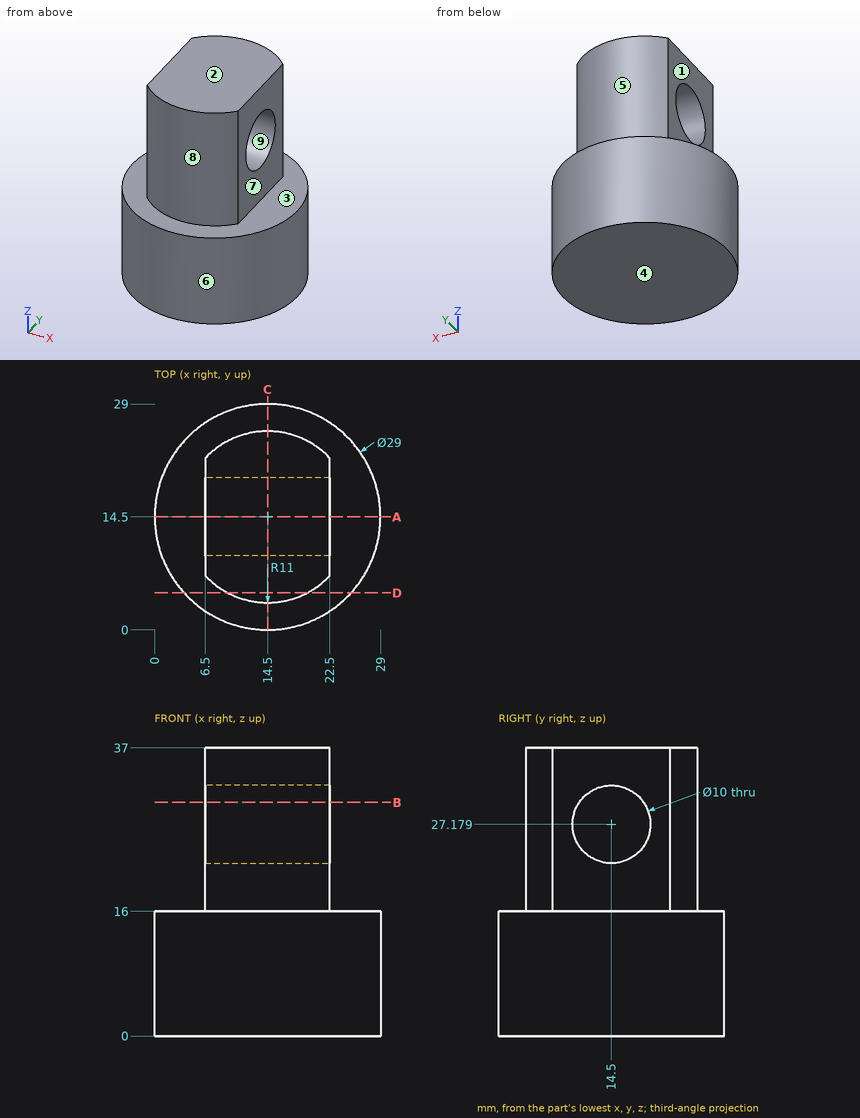
Geometry check sheet. Reference: drawing and pictorial views, mm from the part's lowest x, y, z. A direction names the side the tool comes from. Coordinates: 2 decimals unless noted, no trailing zeros. Loops run counter-clockwise (first coordinate to the right, second up) from the corner with the lowest first, then second, coordinate; pieces in that order, holes last.
1) Sectioned sample at B-B (z = 30). Record the boundary of the cut face in (x, y), and give its area (3 significant figures).
2) Release check for a two-part mould opening along Y. For the marked faces 6, 7, 8 and 9 record: released by +Y, released by -Y, zero draft, split by the parting line, or undercut.
3) Access from +Z, -Z, +X, -X, +Y, -Y to the whole of each face (thin tool, end or side, straight path). Record for the marked faces 1, 2, 3, 4 and 5.
4) Material ranges on probe 1 along Z at (x, y) = (14.75, 14.5); probe 2 along Z at (x, y) = (12, 2); probe 3 along X at (y, z) = (8.5, 18), recorded low to high.
5) Gauge pin test, flat ends, axial feed: pin 1 (2 mm diameter, centred on x = 10.5, z = 9.5, fed in from -Y); pin 2 (4 mm diameter, centred on x = 24.5, z = 5, fed in from -Y); pin 3 (3 mm diameter, centred on y = 11, z = 13, fed in from +X). Record the tip position at first contact, or that the pin passes through.
6) Sectioned sample at D-D (y = 4.75). Record the boundary of the cut face in (x, z).
7) Sectioned sample at C-C (x = 14.5). Record the boundary of the cut face in (y, z).
8) Sectioned sample at A-A (y = 14.5). Record the boundary of the cut face in (x, z), and give its area (3 significant figures).
Check sheet entries:
1. outline: (6.5, 6.95) arc R11 ccw to (22.5, 6.95) - (22.5, 10.37) - (6.5, 10.37) - close; (6.5, 18.63) - (22.5, 18.63) - (22.5, 22.05) arc R11 ccw to (6.5, 22.05) - close
1. area: 186 mm2
2. face 6: split by the parting line
2. face 7: zero draft
2. face 8: released by -Y
2. face 9: undercut
3. face 1: +Z, -X, +Y, -Y
3. face 2: +Z, +X, -X, +Y, -Y
3. face 3: +Z
3. face 4: -Z, +X, -X, +Y, -Y
3. face 5: +Z, +Y
4. probe 1: z = 0 to 22.18, 32.18 to 37
4. probe 2: z = 0 to 16
4. probe 3: x = 6.5 to 22.5
5. pin 1: stops at y = 0.31
5. pin 2: stops at y = 2.41
5. pin 3: stops at x = 28.86
6. outline: (3.77, 0) - (25.23, 0) - (25.23, 16) - (19.59, 16) - (19.59, 37) - (9.41, 37) - (9.41, 16) - (3.77, 16) - close
7. outline: (0, 0) - (29, 0) - (29, 16) - (25.5, 16) - (25.5, 37) - (3.5, 37) - (3.5, 16) - (0, 16) - close; hole circle Ø10 at (14.5, 27.18)
8. outline: (0, 0) - (29, 0) - (29, 16) - (22.5, 16) - (22.5, 22.18) - (6.5, 22.18) - (6.5, 16) - (0, 16) - close; (6.5, 32.18) - (22.5, 32.18) - (22.5, 37) - (6.5, 37) - close
8. area: 640 mm2
